Input: part model. Units: mm. Frame: model coordinates. A direction names the side the tool comes from. Give positions to 0.01 mm unless a question says otherwise; leave off trailing zeros. Loops run counter-clockwise (first coordinate to the right, second up) from the corner with the lowest first, then second, coordinate; pieces in that order, holes last. Notation, with made-up numbers: (19, 69.5) - (29, 69.5) arc R29 cw to (29, 89.5) - close; hole circle Ø8 at (32, -31). An arc over 180 degrees is marked (long way). One line per item, written item: value.
from build123d import *

# Parameters (mm, degrees)
BOSS_EXTRUDE1_DEPTH = 5
FILLET1_R           = 10
FILLET2_R           = 5


with BuildPart() as part:
    # Sketch1 → Boss-Extrude1 (new body)
    with BuildSketch(Plane.XY):
        Polygon((-18.484799863, 5), (-21.984799863, 5), (-21.984799863, 0), (-26.984799863, 0), (-26.984799863, 5), (-26.984799863, 21.097384909), (-11.984799863, 21.097384909), (-11.984799863, 5), (-15.484799863, 5), (-15.484799863, 8), (-14.384799863, 8), (-14.384799863, 10.3), (-15.484799863, 10.3), (-15.484799863, 15), (-18.484799863, 15), (-18.484799863, 10.3), (-19.584799863, 10.3), (-19.584799863, 8), (-18.484799863, 8), align=None)
    extrude(amount=BOSS_EXTRUDE1_DEPTH)

    # Fillet1
    fillet1_edges = [part.edges().sort_by_distance(p)[0] for p in [
        (-26.984799863, 21.097384909, 2.5),
    ]]
    fillet(fillet1_edges, radius=FILLET1_R)

    # Fillet2
    fillet2_edges = [part.edges().sort_by_distance(p)[0] for p in [
        (-11.984799863, 21.097384909, 2.5),
    ]]
    fillet(fillet2_edges, radius=FILLET2_R - 0.0001)  # a hair under: the kernel refuses the full size


solid = part.part
Item 1: Section D-D, the plane y = 4.5. Output: boundary loops of the cut face in (x, z).
Verdict:
outline: (-26.98, 0) - (-21.98, 0) - (-21.98, 5) - (-26.98, 5) - close
Item 2: Section A-A, the plane y = 7.75. Output: boundary loops of the cut face in (x, z).
Verdict:
outline: (-26.98, 0) - (-18.48, 0) - (-18.48, 5) - (-26.98, 5) - close; (-15.48, 0) - (-11.98, 0) - (-11.98, 5) - (-15.48, 5) - close
Item 3: Draft query along Y for faces 1 (the face through (-14.385, 9, 2)), 2 (the face through (-20, 5, 2)), 3 (the face through (-19, 11, 0)). Return one class per face: pulls with the +Y half, pulls with the -Y half, needs draft (parallel to the pull), parting line crosses it, or undercut.
Verdict:
face 1: undercut
face 2: pulls with the -Y half
face 3: needs draft
Item 4: Section C-C, the plane y = 13.25. Output: boundary loops of the cut face in (x, z), and give its area (3 significant figures).
Verdict:
outline: (-26.75, 0) - (-18.48, 0) - (-18.48, 5) - (-26.75, 5) - close; (-15.48, 0) - (-11.98, 0) - (-11.98, 5) - (-15.48, 5) - close
area: 58.8 mm^2
Item 5: Access query for faces 4 (the face through (-15, 8, 2)), 5 (the face through (-17, 15, 2)), 6 (the face through (-14, 5, 2)). Directions: +Z, -Z, +X, -X, +Y, -Y. A direction counts if a zero-diameter tool reaches every point of the face in a straight line with its end or side. Return the directions, or none.
Verdict:
face 4: +Z, -Z
face 5: +Z, -Z, -Y
face 6: +Z, -Z, +X, -Y
Item 6: Material intervals for L1, parallel to X at y = 9.75, z = 3.2; L2, parallel to X at y = 6.5, z = 0.75; L3, parallel to Y at x = -18.75, z = 3.75, sorted ascending.
Verdict:
L1: x = -26.98 to -19.58, -14.38 to -11.98
L2: x = -26.98 to -18.48, -15.48 to -11.98
L3: y = 5 to 8, 10.3 to 20.94
Item 7: Pin query (flat end, axial travel): P1, Ø3, axis at x = -24, z = 1, coming from the +Y side; P2, Ø1.2, axis at x = -15, z = 2.5, coming from the +Y side; P3, Ø1.5, axis at x = -17, z = 2, coming from the -Y side. Return the tip coordinate at first contact, or that it passes through.
Verdict:
P1: stops at y = 19.44
P2: stops at y = 20.9
P3: stops at y = 15
